from build123d import *

# Parameters (mm, degrees)
SKETCH_1_R          = 21
SKETCH_1_R_2        = 8
EXTRUDE_1_DEPTH     = 5
HOLE_WIZARD_M41_D   = 4.5
SKETCH_4_R          = 9
CUT_EXTRUDE_1_DEPTH = 0.8


with BuildPart() as part:
    # Эскиз1 → Бобышка-Вытянуть1 (new body)
    with BuildSketch(Plane.XY):
        Circle(SKETCH_1_R)
        Circle(SKETCH_1_R_2, mode=Mode.SUBTRACT)
    extrude(amount=EXTRUDE_1_DEPTH)

    # Отверстие с зазором M41 (through all)
    with Locations(Plane.XY.offset(5)):
        with Locations((0, 16), (-16, 0), (0, -16), (16, 0)):
            Hole(HOLE_WIZARD_M41_D / 2)

    # Эскиз4 → Вырез-Вытянуть1 (cut)
    with BuildSketch(Plane.XY.offset(5)):
        Circle(SKETCH_4_R)
    extrude(amount=-CUT_EXTRUDE_1_DEPTH, mode=Mode.SUBTRACT)


solid = part.part
Source: CAD feature listing. Evaluate the final solid. Frame: model axes, mm. A direction names the side the tool comes from. Give positions to 0.01 mm unless a question says otherwise; leave off trailing zeros. Loops run counter-clockwise (first coordinate to the right, second up) from the corner with the lowest first, then second, coordinate; pieces in that order, holes last. Notation, with made-up numbers: (35.25, 19) -> (39.25, 19) arc R11 ccw to (39.25, 27) -> close; hole circle Ø7 at (66, 53). An arc over 180 degrees is marked (long way). Use a Markdown table: item, result. Add a question column.
1) Section query A-A, the plane x = 0. Return the cut outline in (y, z), then the cut area to 3 significant figures.
2) Line query: line 1 along X through (y, z) = (6, 3.65); line 2 along X through (y, z) = (6.5, 1.15); line 3 along Y through (x, z) = (7, 1.7). Output: solid intervals per line, ascending. Write a range as [from, to].
3) Section query C-C, the plane z = 1.95. Return the cut outline in (x, y).
4) Pull-direction query (Y, two-part tool) for faces 3 (the face through (-18.146, 0.676, 2.465)), 4 (the face through (9, 0, 0)), 5 (the face through (20.03, 6.31, 2.46)), 6 (the face through (0.488, 13.804, 2.465)); classes: +Y half, -Y half, draft (parallel to the pull), parting line (faces both ways), or undercut.
5) Section query B-B, the plane y = 16. Return the cut outline in (x, z), then the cut area to 3 significant figures.
6) First-contact query: pin 1 (2.5 mm diameter, centred on x = 0, y = -16, fed in from +Z); pin 2 (2 mm diameter, centred on x = -14.5, z = 1, fed in from +Y). Flat tips, straight axial feed; report the tip coordinate or a pass-through.
7) Reachability of faces 1 (the face through (-1.172, 8.923, 4.606)), 2 (the face through (9, -4, 5)) from +Z, -Z, +X, -X, +Y, -Y: full face, straight path, thin tool, end or side. Return the list, or none.
Numbers:
| question | item | result |
|---|---|---|
| 1 | outline | (-21, 0) -> (-18.25, 0) -> (-18.25, 5) -> (-21, 5) -> close; (-13.75, 0) -> (-8, 0) -> (-8, 4.2) -> (-9, 4.2) -> (-9, 5) -> (-13.75, 5) -> close; (8, 0) -> (13.75, 0) -> (13.75, 5) -> (9, 5) -> (9, 4.2) -> (8, 4.2) -> close; (18.25, 0) -> (21, 0) -> (21, 5) -> (18.25, 5) -> close |
| 1 | area | 83.4 mm2 |
| 2 | line 1 | x = [-20.12, -5.29], [5.29, 20.12] |
| 2 | line 2 | x = [-19.97, -4.66], [4.66, 19.97] |
| 2 | line 3 | y = [-19.8, -3.87], [3.87, 19.8] |
| 3 | outline | circle Ø42 at (0, 0); hole circle Ø4.5 at (-16, 0); hole circle Ø16 at (0, 0); hole circle Ø4.5 at (0, -16); hole circle Ø4.5 at (0, 16); hole circle Ø4.5 at (16, 0) |
| 4 | face 3 | undercut |
| 4 | face 4 | draft |
| 4 | face 5 | parting line |
| 4 | face 6 | undercut |
| 5 | outline | (-13.6, 0) -> (-2.25, 0) -> (-2.25, 5) -> (-13.6, 5) -> close; (2.25, 0) -> (13.6, 0) -> (13.6, 5) -> (2.25, 5) -> close |
| 5 | area | 114 mm2 |
| 6 | pin 1 | passes through |
| 6 | pin 2 | stops at y = 16.09 |
| 7 | face 1 | +Z |
| 7 | face 2 | +Z, +X, -X, +Y, -Y |
